Part model, mm, in its own coordinate system. Face numbers are marked on the shaded views. A direction names the side the tool comes from. Coordinates: 2 decimals unless noted, no trailing zeros. Order: outer loops, then holes, each group sorted by start corner. A loop starts at its lowest first (then second) coordinate and runs counter-clockwise, first axis right, second up.
1) Cut at C-C (x = -8). List the corners of the cut face in (y, z), and give its area (3 significant figures).
2) Wall check: L1, parallel to X at y = -7.75, z = -19.5; L2, parallel to Z at x = -10, y = -9; L3, parallel to Z at x = 13, y = 9.25. Give the ranges that are in metal, low to high.
3) Cut at B-B (z = 45). List the corners of the cut face in (x, y).
4) Pin check, flat tips, straight feed: pin 1 Ø10 at (y, z) = (-1, -25.5) entering from -X; pin 2 Ø8 at (x, y) = (-8.5, -6) entering from -Z; pin 3 Ø2.5 at (x, z) = (14, -99.5) entering from -Y. Stop position of each tip, or through.
5) Cut at A-A (y = 7.5). List the corners of the cut face in (x, z).
6) Tool access for the marked faces 1 and 2: list every direction of +Z, -Z, +X, -X, +Y, -Y with a clear straight run to the whole face (end or side of a thin tool).
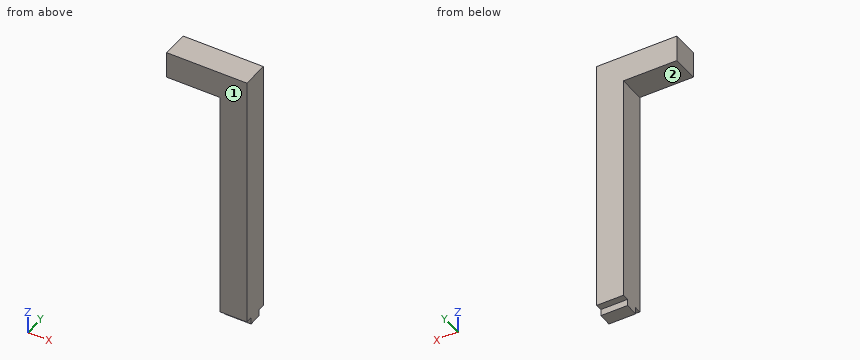
```python
from build123d import *

# Parameters (mm, degrees)
F0_W     = 20
F0_H     = 195
F1_DEPTH = 20
F2_W     = 20
F2_H     = 10
F3_DEPTH = 5
F4_W     = 20
F4_H     = 20
F5_DEPTH = 40


with BuildPart() as f1:
    # F0 (on Right) → F1 (new body)
    with BuildSketch(Plane.YZ):
        Rectangle(F0_W, F0_H)
    extrude(amount=F1_DEPTH)

    # F2 (on face) → F3 (join)
    with BuildSketch(Plane(origin=(0, 0, -97.5), x_dir=(1, 0, 0), z_dir=(0, 0, -1))):
        with Locations((10, 0)):
            Rectangle(F2_W, F2_H)
    extrude(amount=F3_DEPTH)

    # F4 (on face) → F5 (join)
    with BuildSketch(Plane(origin=(0, 0, 0), x_dir=(0, -1, 0), z_dir=(-1, 0, 0))):
        with Locations((0, 87.5)):
            Rectangle(F4_W, F4_H)
    extrude(amount=F5_DEPTH)


solid = f1.part
```
Geometry check:
1. outline: (-10, 77.5) - (10, 77.5) - (10, 97.5) - (-10, 97.5) - close
1. area: 400 mm2
2. L1: x = 0 to 20
2. L2: z = 77.5 to 97.5
2. L3: z = -97.5 to 97.5
3. outline: (0, -10) - (20, -10) - (20, 10) - (0, 10) - close
4. pin 1: stops at x = 0
4. pin 2: stops at z = 77.5
4. pin 3: stops at y = -5
5. outline: (-40, 77.5) - (0, 77.5) - (0, -97.5) - (20, -97.5) - (20, 97.5) - (-40, 97.5) - close
6. face 1: +Z, -Z, +X, -X, -Y
6. face 2: -Z, -X, +Y, -Y
